from build123d import *

# Parameters (mm, degrees)
F1_DEPTH = 12.7
F2_R     = 4.566198
F2_R_2   = 4.930932
F3_DEPTH = 12.7


with BuildPart() as f1:
    # F0 (on Front) → F1 (new body, symmetric)
    with BuildSketch(Plane.XZ):
        with BuildLine():
            Line((47.752, 38.1), (47.752, 76.2))
            Line((47.752, 76.2), (-47.498, 76.2))
            Line((-47.498, 76.2), (-47.498, 38.1))
            Line((-47.498, 38.1), (-18.904509, 38.1))
            ThreePointArc((-18.904509, 38.1), (0, 57.004509), (18.904509, 38.1))
            Line((18.904509, 38.1), (47.752, 38.1))
        make_face()
        with BuildLine():
            Line((47.752, 0), (47.752, 38.1))
            Line((47.752, 38.1), (18.904509, 38.1))
            ThreePointArc((18.904509, 38.1), (0, 19.195491), (-18.904509, 38.1))
            Line((-18.904509, 38.1), (-47.498, 38.1))
            Line((-47.498, 38.1), (-47.498, 0))
            Line((-47.498, 0), (47.752, 0))
        make_face()
    extrude(amount=F1_DEPTH, both=True)

    # F2 (on face) → F3 (cut, symmetric)
    with BuildSketch(Plane.XY.offset(76.2)):
        with Locations((-38.714517, 0)):
            Circle(F2_R)
        with Locations((37.485483, 0)):
            Circle(F2_R_2)
    extrude(amount=F3_DEPTH, both=True, mode=Mode.SUBTRACT)


solid = f1.part
Part model, mm, in its own coordinate system. A direction names the side the tool comes from. Round coordinates to 2 decimals unless told otherwise and drop trailing zeros. Write each loop counter-clockwise with the first axis right and the second up, starting at its lowest first coordinate (ties: lowest second). Pieces come first, ordered by that corner, then holes. Notation, with made-up numbers: (8.5, 62.5) - (51.5, 62.5) arc R17 ccw to (51.5, 77.5) - close; hole circle Ø2 at (-17, -2). An arc over 180 degrees is marked (long way). Use CSV: the item, a comma, the result in double quotes.
Item 1: Wall check: L1, parallel to X at y = 0.25, z = 38.1; L2, parallel to X at y = -2, z = 67.5; L3, parallel to Z at x = 0, y = 0. Give the ranges that are in metal, low to high.
Results list:
L1,"x = -47.5 to -18.9, 18.9 to 47.75"
L2,"x = -47.5 to -42.82, -34.61 to 32.98, 41.99 to 47.75"
L3,"z = 0 to 19.2, 57 to 76.2"
Item 2: Tool access for faces 5 (the cylindrical face through (-43.276, 0.201, 69.939)), 6 (the flat face through (-47.498, 0, 39)): list every direction of +Z, -Z, +X, -X, +Y, -Y with a clear straight run to the whole face (end or side of a thin tool).
Results list:
face 5,"+Z"
face 6,"+Z, -Z, -X, +Y, -Y"
Item 3: Pull direction Y, two halves, no side cores. Call faces 1 (the flat face through (-39, 0, 63.5)), 2 (the flat face through (10, 12.7, 56)), 3 (the flat face through (47.752, 0, 38)), 4 (the flat face through (10, -12.7, 56)): pulls with the +Y half, pulls with the -Y half, needs draft (parallel to the pull), parting line crosses it, or undercut.
Results list:
face 1,"undercut"
face 2,"pulls with the +Y half"
face 3,"needs draft"
face 4,"pulls with the -Y half"
Item 4: Slice it at B-B, the plane y = 0. Write the cut outline in (x, z), then the cut area to 3 significant figures.
Results list:
outline,"(-47.5, 0) - (47.75, 0) - (47.75, 76.2) - (42.42, 76.2) - (42.42, 63.5) - (32.55, 63.5) - (32.55, 76.2) - (-34.15, 76.2) - (-34.15, 63.5) - (-43.28, 63.5) - (-43.28, 76.2) - (-47.5, 76.2) - close; hole circle Ø37.81 at (0, 38.1)"
area,"5,890 mm²"
Item 5: Slice it at A-A, the plane z = 38.1. Write the cut outline in (x, y), then the cut area to 3 significant figures.
Results list:
outline,"(-47.5, -12.7) - (-18.9, -12.7) - (-18.9, 12.7) - (-47.5, 12.7) - close; (18.9, -12.7) - (47.75, -12.7) - (47.75, 12.7) - (18.9, 12.7) - close"
area,"1,460 mm²"
Item 6: Slice it at D-D, the plane z = 68.5. Write the cut outline in (x, y), then the cut area to 3 significant figures.
Results list:
outline,"(-47.5, -12.7) - (47.75, -12.7) - (47.75, 12.7) - (-47.5, 12.7) - close; hole circle Ø9.13 at (-38.71, 0); hole circle Ø9.86 at (37.49, 0)"
area,"2,280 mm²"
Item 7: Flat gauge pin, fed straight in: P1, Ø8, axis at x = -38.71, y = 0, coming from the +Z side. Where does the tip first touch, or does it go through?
Results list:
P1,"stops at z = 63.5"
Item 8: Slice it at C-C, the plane x = 0. Write the cut outline in (y, z), then the cut area to 3 significant figures.
Results list:
outline,"(-12.7, 0) - (12.7, 0) - (12.7, 19.2) - (-12.7, 19.2) - close; (-12.7, 57) - (12.7, 57) - (12.7, 76.2) - (-12.7, 76.2) - close"
area,"975 mm²"
